Check sheet for the modelled part. Datum: model origin and axes. Units: mm. A direction names the side the tool comes from. Round coordinates to 2 decimals unless told otherwise and drop trailing zeros. Loops run counter-clockwise (first coordinate to the right, second up) from the corner with the lowest first, then second, coordinate; pieces in that order, holes last. Notation, with made-up numbers: (63.5, 71) - (68.5, 71) arc R23 ccw to (68.5, 107) - close; hole circle Ø3 at (-21, -2). An arc over 180 degrees is marked (long way). Answer in a Markdown table with one row per item. Add a question column.
(1) Thickness scan on line 1 along X through (y, z) = (17.5, 25); line 2 along Z through (x, y) = (85, 7.5); line 3 along Z through (x, y) = (102.5, 14.5). Record the ranges inside material, lowest first.
(2) Cross-section at C-C on y = 24. Enter the section's corners in (x, z), then the cut area to 3 significant figures.
(3) Cross-section at D-D on x = 123.5. Enter the section's corners in (y, z), then the cut area to 3 significant figures.
(4) Gauge pin test, flat ends, axial feed: pin 1 (25 mm diameter, centred on x = 23.5, z = 23, fed in from +Y); pin 2 (8 mm diameter, centred on y = 27.5, z = 36.5, fed in from -X). Record the tip position at first contact, or that the pin passes through.
(5) Cross-section at B-B on z = 7.5. Enter the section's corners in (x, y).
(6) Access from +Z, -Z, +X, -X, +Y, -Y to the whole of each face (thin tool, end or side, straight path). Record for faces 4 (the flat face through (193.312, 8.256, 24.65)), 5 (the flat face through (-192.164, 8.984, 24.664)).
(7) Cross-section at A-A on y = 6.5. Enter the section's corners in (x, z).
(8) Mould release check, pull along X, two halves, no side actions. Record for faces 1 (the flat face through (-83, 31.5, 23)), 2 (the flat face through (-2, 1, 25)), 3 (the flat face through (-194.19, 8.49, 24.65)): +X half, -X half, draft (parallel to the pull), parting line (faces both ways), or undercut.
from build123d import *

# Parameters (mm, degrees)
BOSS_EXTRUDE1_DEPTH = 50
SHELL1_T            = -1
SKETCH2_R           = 2.5
CUT_EXTRUDE1_DEPTH  = 50
SKETCH3_R           = 5
SKETCH3_R_2         = 2.5
BOSS_EXTRUDE2_DEPTH = 30.5


with BuildPart() as part:
    # Sketch1 → Boss-Extrude1 (new body)
    with BuildSketch(Plane.XY):
        Polygon((-162.5, 0), (162.5, 0), (225, 16.746824527), (-225, 16.746824527), align=None)
    extrude(amount=BOSS_EXTRUDE1_DEPTH)

    # Shell1
    shell1_openings = [part.faces().sort_by_distance(p)[0] for p in [
        (0, 16.746824527, 25),
    ]]
    offset(amount=SHELL1_T, openings=shell1_openings, kind=Kind.INTERSECTION)

    # Sketch2 → Cut-Extrude1 (cut)
    with BuildSketch(Plane.XZ):
        with Locations(Location((-85, 25, 0), (0, 0, 270))):
            Circle(SKETCH2_R)
        with Locations(Location((85, 25, 0), (0, 0, 270))):
            Circle(SKETCH2_R)
    extrude(amount=-CUT_EXTRUDE1_DEPTH, mode=Mode.SUBTRACT)

    # Sketch3 → Boss-Extrude2 (add)
    # profile 1 of 2: a face of its own
    with BuildSketch(Plane(origin=(0, 1, 0), x_dir=(1, 0, 0), z_dir=(0, 1, 0))):
        with Locations(Location((-85, -25, 0), (0, 0, 90))):
            Circle(SKETCH3_R)
        with Locations(Location((-85, -25, 0), (0, 0, 90))):
            Circle(SKETCH3_R_2, mode=Mode.SUBTRACT)
    # profile 2 of 2: a face of its own
    with BuildSketch(Plane(origin=(0, 1, 0), x_dir=(1, 0, 0), z_dir=(0, 1, 0))):
        with Locations(Location((85, -25, 0), (0, 0, 90))):
            Circle(SKETCH3_R)
        with Locations(Location((85, -25, 0), (0, 0, 90))):
            Circle(SKETCH3_R_2, mode=Mode.SUBTRACT)
    extrude(amount=BOSS_EXTRUDE2_DEPTH)


solid = part.part
Answers:
| question | item | result |
|---|---|---|
| 1 | line 1 | x = -90 to -87.5, -82.5 to -80, 80 to 82.5, 87.5 to 90 |
| 1 | line 2 | z = 0 to 1, 20 to 22.5, 27.5 to 30, 49 to 50 |
| 1 | line 3 | z = 0 to 1, 49 to 50 |
| 2 | outline | circle Ø10 at (-85, 25); circle Ø10 at (85, 25); hole circle Ø5 at (-85, 25); hole circle Ø5 at (85, 25) |
| 2 | area | 118 mm^2 |
| 3 | outline | (0, 0) - (16.75, 0) - (16.75, 1) - (1, 1) - (1, 49) - (16.75, 49) - (16.75, 50) - (0, 50) - close |
| 3 | area | 81.5 mm^2 |
| 4 | pin 1 | stops at y = 1 |
| 4 | pin 2 | passes through |
| 5 | outline | (-225, 16.75) - (-162.5, 0) - (162.5, 0) - (225, 16.75) - (221.14, 16.75) - (162.37, 1) - (-162.37, 1) - (-221.14, 16.75) - close |
| 6 | face 4 | +Z, -Z, +X, -Y |
| 6 | face 5 | +Y |
| 7 | outline | (-186.76, 0) - (186.76, 0) - (186.76, 50) - (-186.76, 50) - close; circle Ø10 at (-85, 25); circle Ø10 at (85, 25); hole (-182.89, 1) - (182.89, 1) - (182.89, 49) - (-182.89, 49) - close; hole circle Ø5 at (-85, 25); hole circle Ø5 at (85, 25) |
| 8 | face 1 | draft |
| 8 | face 2 | undercut |
| 8 | face 3 | -X half |
